The model under review builds one solid part; all positions refer to its coordinate system, in mm. A direction names the side the tool comes from. Coordinates: 2 decimals unless noted, no trailing zeros. Loops run counter-clockwise (first coordinate to the right, second up) from the corner with the lowest first, then second, coordinate; pieces in that order, holes last. Notation, with made-up numbers: M 13,-11.75 L 63,-11.75 A16 cw 63,7.25 Z; hole C -39,-3.5 d5. An arc over 180 degrees is marked long. Use CSV: the item, a comma, the result in double quotes. Start each with the question number.
1. Add section A-A, the plane x = -1.1. Write out the cut boundary in (y, z), then the cut area to 4 significant figures.
2. Tool access review of faces 1 (the flat face through (1, 7, -12.5)), 2 (the flat face through (0, 7, 10.5)): name each direction out of +Z, -Z, +X, -X, +Y, -Y from which nothing blocks a thin tool from reaching the whole face with its end or side.
3. Add section D-D, the plane z = 12. Write out the cut boundary in (x, y), then the cut area to 3 significant figures.
4. For L1, parallel to Z at x = -0.45, y = 8; L2, parallel to X at y = 11.5, z = -9.5; L3, parallel to Y at x = -2.1, z = 8, list the stretches that pass through material, from the lowest coordinate up.
5. Add section B-B, the plane z = -5.5. Write out the cut boundary in (x, y), then the cut area to 3 significant figures.
6. Draft analysis for pull direction Z (two halves, no side actions). For faces 3 (the flat face through (2, 14, -1)), 4 (the flat face through (0, 9, 26.5)), 5 (the flat face through (-1.5, 7, 0)), 6 (the flat face through (0, 7, -10.5)), state which applies: +Z half, -Z half, draft (parallel to the pull), parting line (faces both ways), or undercut.
7. Add section C-C, the plane y = 10. Write out the cut boundary in (x, z), then the cut area to 3 significant figures.
from build123d import *

# Parameters (mm, degrees)
EXTRUDE_2_DEPTH = 14
SKETCH_3_W      = 6
SKETCH_3_H      = 16
EXTRUDE_3_DEPTH = 5
CHAMFER_1_SIZE  = 5


with BuildPart() as part:
    # Эскиз1 → Бобышка-Вытянуть2 (new body)
    with BuildSketch(Plane(origin=(0, 0, 0), x_dir=(1, 0, 0), z_dir=(0, 1, 0))):
        Polygon((-2.5, -26.5), (-1.5, -26.5), (3.5, -26.5), (3.5, -12.5), (3.5, -7.973274813), (3.5, 12.5), (-1.5, 12.5), (-2.5, 12.5), align=None)
        Polygon((1.5, -10.5), (-1.5, -10.5), (-1.5, -5.357142857), (-1.5, 5.357142857), (-1.5, 10.5), (1.5, 10.5), align=None, mode=Mode.SUBTRACT)
    extrude(amount=EXTRUDE_2_DEPTH)

    # Эскиз3 → Бобышка-Вытянуть3 (add)
    with BuildSketch(Plane(origin=(0, 14, 0), x_dir=(1, 0, 0), z_dir=(0, 1, 0))):
        with Locations((0.5, -18.5)):
            Rectangle(SKETCH_3_W, SKETCH_3_H)
    extrude(amount=EXTRUDE_3_DEPTH)

    # Фаска1
    chamfer_1_edges = [part.edges().sort_by_distance(p)[0] for p in [
        (0.5, 19, 10.5),
    ]]
    chamfer(chamfer_1_edges, length=CHAMFER_1_SIZE)


solid = part.part
Computed:
1,outline,"M 0,-12.5 L 14,-12.5 L 14,-10.5 L 0,-10.5 Z; M 0,10.5 L 14,10.5 L 19,15.5 L 19,26.5 L 0,26.5 Z"
1,area,"319.5 mm^2"
2,face 1,"-Z, +X, -X, +Y, -Y"
2,face 2,"+Y, -Y"
3,outline,"M -2.5,0 L 3.5,0 L 3.5,15.5 L -2.5,15.5 Z"
3,area,"93.0 mm^2"
4,L1,"z = -12.5 to -10.5, 10.5 to 26.5"
4,L2,"x = -2.5 to -1.5, 1.5 to 3.5"
4,L3,"y = 0 to 14"
5,outline,"M -2.5,0 L -1.5,0 L -1.5,14 L -2.5,14 Z; M 1.5,0 L 3.5,0 L 3.5,14 L 1.5,14 Z"
5,area,"42.0 mm^2"
6,face 3,"draft"
6,face 4,"+Z half"
6,face 5,"undercut"
6,face 6,"undercut"
7,outline,"M -2.5,-12.5 L 3.5,-12.5 L 3.5,26.5 L -2.5,26.5 Z; hole M -1.5,-10.5 L 1.5,-10.5 L 1.5,10.5 L -1.5,10.5 Z"
7,area,"171 mm^2"
